The figure shows three views and two pictorial views of one solid part (mm, origin at its lowest corner). Answer the questions. A direction names the side the tool comes from. Give positions to 0.01 mm unless a question says otherwise; leave off trailing zeros. Write each loop counter-clockwise with the first axis right and the second up, starting at its lowest first coordinate (ties: lowest second). Pieces come first, ordered by that corner, then holes. Notation, with made-up numbers: (26, -27.75) - (60, -27.75) arc R7 cw to (60, -15.75) - close; hole circle Ø10 at (30.5, 48.25). An arc over 180 degrees is marked (long way). One line per question, with ' | ' between items. Start each with the question number.
1. A cutting plane is placed at D-D (x = 3.5). Determine the outline of the cut face in (y, z).
2. Find the intervals of material crossed by L1, parallel to Y at x = 8.5, z = 0.7 (1 decimal); L2, parallel to Y at x = 8, z = 2.8 (1 decimal); L3, parallel to X at y = 29, z = 1.3 (1 decimal), in increasing order. Write a range as from..to.
3. Given P1, Ø1, axis at y = 20.5, z = 1.5, coming from the -X side; P2, Ø1.5, axis at x = 2, z = 0.5, coming from the +Y side (1 decimal); P3, Ø1.5, axis at x = 7.55, y = 37.37, coming from the -Z side; P4, Ø4, axis at x = 4.44, y = 3.51, coming from the -Z side, each flat-ended and moving along its own axis, determine where each tip first touches the part or whether it passes through.
4. A cutting plane is placed at A-A (z = 2.15). State how many separate pieces and enclosed holes the cut face has, then the cut area to 3 significant figures.
5. For the marked faces 1 and 2, determine the directions among +Z, -Z, +X, -X, +Y, -Y from which every point of the face is accessible in a straight line to the end or side of a thin tool.
6. A cutting plane is placed at C-C (y = 29). Determine the outline of the cut face in (x, z) (1 decimal), then the cut area to 3 significant figures.
7. A cutting plane is placed at B-B (x = 8.25). Determine the outline of the cut face in (y, z).
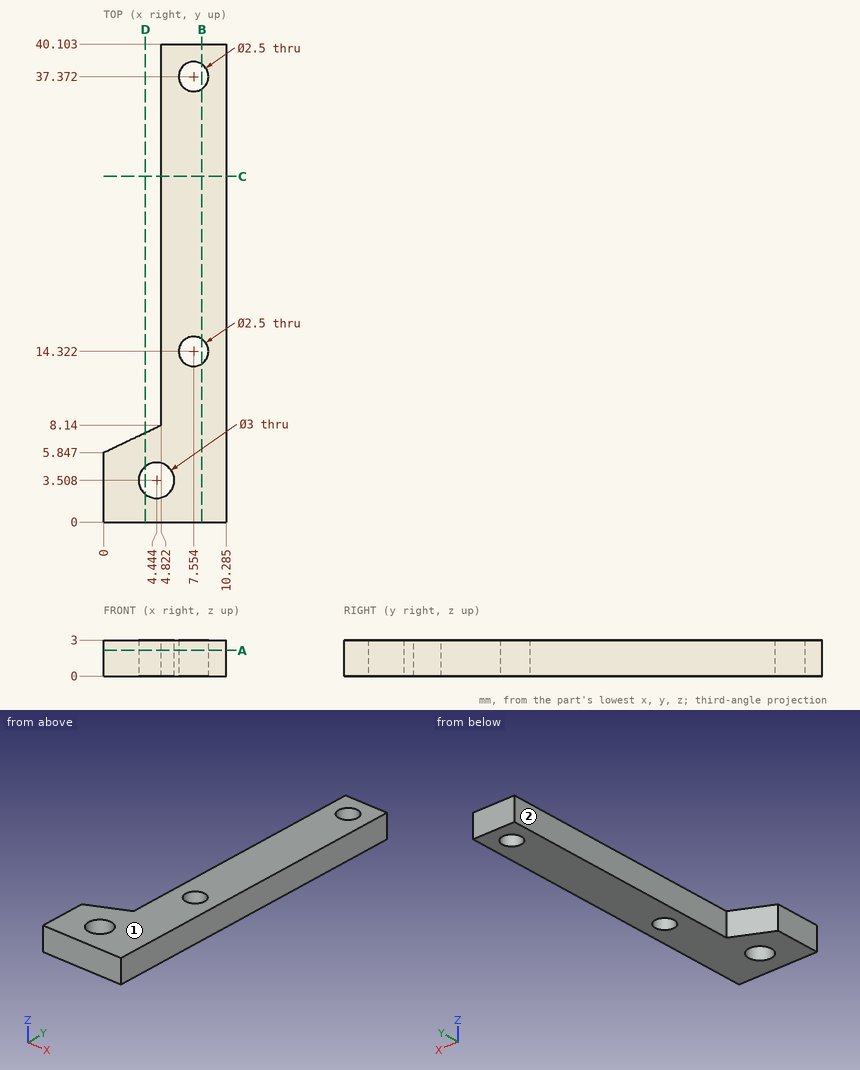
Determined:
1) outline: (0, 0) - (2.34, 0) - (2.34, 3) - (0, 3) - close; (4.67, 0) - (7.51, 0) - (7.51, 3) - (4.67, 3) - close
2) L1: 0..13.5, 15.1..36.6, 38.2..40.1 | L2: 0..13.2, 15.5..36.2, 38.5..40.1 | L3: 4.8..10.3
3) P1: x = 4.82 | P2: y = 7.2 | P3: through | P4: z = 0
4) separate pieces: 1 | enclosed holes: 3 | area: 236 mm2
5) face 1: +Z, +X, -X, +Y, -Y | face 2: +Z, -Z, -X, +Y
6) outline: (4.8, 0) - (10.3, 0) - (10.3, 3) - (4.8, 3) - close | area: 16.4 mm2
7) outline: (0, 0) - (13.28, 0) - (13.28, 3) - (0, 3) - close; (15.36, 0) - (36.33, 0) - (36.33, 3) - (15.36, 3) - close; (38.41, 0) - (40.1, 0) - (40.1, 3) - (38.41, 3) - close
